Geometry check sheet. Reference: the model listing, model coordinates, mm. A direction names the side the tool comes from. Round coordinates to 2 decimals unless told otherwise and drop trailing zeros. Loops run counter-clockwise (first coordinate to the right, second up) from the corner with the lowest first, then second, coordinate; pieces in that order, holes last.
Autodesk Inventor part; units mm, degrees
ref_plane "YZ Plane" through (0, 0, 0) normal (1, 0, 0) x (0, 1, 0)
ref_plane "XZ Plane" through (0, 0, 0) normal (0, 1, 0) x (-1, 0, 0)
ref_plane "XY Plane" through (0, 0, 0) normal (0, 0, 1) x (1, 0, 0)
sketch "Эскиз1" plane through (0, 0, 0) normal (0, 0, 1) x (1, 0, 0)
  line L0 (0, 0) -> (345, 0)
  line L1 (345, 0) -> (345, 20)
  line L2 (345, 20) -> (280, 20)
  line L3 (0, 0) -> (0, 22.5)
  line L4 (0, 22.5) -> (50, 22.5)
  line L5 (50, 22.5) -> (70, 22.5)
  line L6 (250, 22.5) -> (230, 22.5)
  line L7 (250, 22.5) -> (265, 18.9255)
  line L8 (265, 18.9255) -> (280, 20)
  line L9 (82.7171, 19.4628) -> (70, 22.5)
  line L10 (50, 22.5) -> (36.6597, 19.4628)
  line L11 (36.6597, 19.4628) -> (0, 19.4628)
  line L12 (230, 22.5) -> (211.3782, 19.4628)
  line L13 (211.3782, 19.4628) -> (82.7171, 19.4628)
  dimension "d0" = 345
  dimension "d1" = 20
  dimension "d2" = 65
  dimension "d5" = 22.5
  dimension "d6" = 50
  dimension "d7" = 20
  dimension "d8" = 20
  dimension "d15" = 30
revolve "Вращение1" add sketch "Эскиз1" angle 360 about axis through (0, 0, 0) along (1, 0, 0) contours L3 L11 L10 L5 L9 L13 L12 L6 L7 L8 L2 L1 L0
thread "Резьба1"
sketch "Эскиз2" plane through (0, 0, 0) normal (-1, 0, 0) x (0, 0, 1)
  circle A0 centre (0, 0) radius 30
  dimension "d12" = 60
extrude "Выдавливание1" add sketch "Эскиз2" along normal blind 1308.008
sketch "Эскиз3" plane through (-1308.008, 0, 0) normal (-1, 0, 0) x (0, 0, 1)
  circle A0 centre (0, 0) radius 22.5
  dimension "d16" = 45
extrude "Выдавливание2" add sketch "Эскиз3" along normal blind 180
sketch "Эскиз4" plane through (0, 0, 0) normal (0, 0, 1) x (1, 0, 0)
  line L0 (-1308.008, 30) -> (-1308.008, -30)
  line L1 (-1488.008, 22.5) -> (-1488.008, -22.5)
  line L2 (-1308.008, -22.5) -> (-1308.008, 22.5)
  line L3 (-1308.008, 0) -> (-1308.008, 20)
  line L4 (-1308.008, 22.5) -> (-1308.008, 20)
  line L5 (-1308.008, 0) -> (-1308.008, -20.008)
  line L6 (-1308.008, -20.008) -> (-1338.008, -20.008)
  line L7 (-1338.008, -20.008) -> (-1340.5, -22.5)
  line L8 (-1340.5, -22.5) -> (-1360.5, -22.5)
  line L9 (-1308.008, -22.5) -> (-1488.008, -22.5)
  line L10 (-1360.5, -22.5) -> (-1362.992, -20.008)
  line L11 (-1366.0081, 27.5) -> (-1366.0081, -27.5)
  line L12 (-1362.992, -20.008) -> (-1388.5, -20.008)
  line L13 (-1388.5, -20.008) -> (-1366.0081, -22.5)
  line L14 (-1308.008, -22.5) -> (-1488.008, -22.5)
  line L15 (-1383, 0) -> (-1400.8637, 0)
  point P0 (-1340.5, -22.5)
  point P1 (-1308.008, -20.008)
  point P2 (-1348.9963, -21.5037)
  dimension "d31" = 30
  dimension "d32" = 135
  dimension "d33" = 20
  dimension "d34" = 135
revolve "Вращение2" cut sketch "Эскиз4" angle 360 about axis through (-1383, 0, 0) along (-1, 0, 0)
chamfer "Фаска1" distance 2 angle 45 1 edges at (-1488.008, 0, -22.5)
thread "Резьба2"
chamfer "Фаска2" distance 2 angle 45 1 edges at (345, -20, 0)
fillet "Сопряжение2" radius 2 3 edges at (-1338.008, 20.008, 0) (-1362.992, 20.008, 0) (-1388.5, 20.008, 0)
properties part number "Шток_CPY" material "Сталь, углеродистая"
1) Sectioned sample at A-A, the plane x = -898. Record the cut outline in (y, z), then the cut area to 3 significant figures.
Report:
outline: circle Ø60 at (0, 0)
area: 2,830 mm2
2) Gauge pin test, flat ends, axial feed: pin 1 (1 mm diameter, centred on x = -1022, z = -2, fed in from +Y); pin 2 (1 mm diameter, centred on x = -29, z = -23.5, fed in from -Y); pin 3 (8 mm diameter, centred on x = -514.5, y = -10, fed in from +Z). Record the tip position at first contact, or that the pin passes through.
Report:
pin 1: stops at y = 29.96
pin 2: stops at y = -19.26
pin 3: stops at z = 29.39
3) Scan lines: line 1 along Z through (x, y) = (208.5, 7); line 2 along Y through (x, z) = (-764, 19.5); line 3 along Z through (x, y) = (-774.5, 20). Record each from-to range of solid material in increasing order.
Report:
line 1: z = -18.16 to 18.16
line 2: y = -22.8 to 22.8
line 3: z = -22.36 to 22.36
4) Access from +Z, -Z, +X, -X, +Y, -Y to the whole of each face (thin tool, end or side, straight path). Record for faces 1 (the face through (80.51, -2.6, -19.82)), 2 (the face through (311.059, -4.336, 19.524)), 3 (the face through (-1487.883, 20.135, -4.471)).
Report:
face 1: none
face 2: +X
face 3: -X
5) Mould release check, pull along X, two halves, no side actions. Record for faces 4 (the face through (345, 0, 0)), 5 (the face through (-1488.008, 0, 0)), 6 (the face through (-1425.168, 19.961, 10.382)), 7 (the face through (0, -20, 0)): +X half, -X half, draft (parallel to the pull), parting line (faces both ways), or undercut.
Report:
face 4: +X half
face 5: -X half
face 6: draft
face 7: undercut
